Part model, mm, in its own coordinate system. Face numbers are marked on the shaded views. A direction names the side the tool comes from. Coordinates: 2 decimals unless noted, no trailing zeros. Write each loop counter-clockwise with the first axis right and the second up, starting at its lowest first coordinate (ties: lowest second). Pieces come first, ordered by that corner, then holes. Notation, with made-up numbers: (25.25, 25) -> (53.25, 25) arc R18 ccw to (53.25, 54) -> close; hole circle Ø1 at (-22, -9.75). An arc over 180 degrees is marked (long way). Write item = value, one per line.
from build123d import *

# Parameters (mm, degrees)
BOSS_EXTRUDE1_DEPTH = 50
FILLET1_R           = 10
SKETCH2_R           = 5
CUT_EXTRUDE1_DEPTH  = 170
SKETCH4_R           = 7.5
CUT_EXTRUDE2_DEPTH  = 10


with BuildPart() as part:
    # Sketch1 → Boss-Extrude1 (new body)
    with BuildSketch(Plane.XY):
        Polygon((0, 0), (0, 275), (160, 275), (160, 0), (150, 0), (150, 265), (10, 265), (10, 0), align=None)
    extrude(amount=BOSS_EXTRUDE1_DEPTH)

    # Fillet1
    fillet1_edges = [part.edges().sort_by_distance(p)[0] for p in [
        (5, 0, 0),
        (0, 275, 25),
        (160, 275, 25),
        (155, 0, 50),
        (5, 0, 50),
        (155, 0, 0),
    ]]
    fillet(fillet1_edges, radius=FILLET1_R)

    # Sketch2 → Cut-Extrude1 (cut)
    with BuildSketch(Plane.ZY):
        with Locations(Location((25, 25, 0), (0, 0, 270))):
            Circle(SKETCH2_R)
    extrude(amount=-CUT_EXTRUDE1_DEPTH, mode=Mode.SUBTRACT)

    # Sketch4 → Cut-Extrude2 (cut)
    with BuildSketch(Plane(origin=(0, 275, 0), x_dir=(1, 0, 0), z_dir=(0, 1, 0))):
        with Locations(Location((75, -25, 0), (0, 0, 270))):
            Circle(SKETCH4_R)
    extrude(amount=-CUT_EXTRUDE2_DEPTH, mode=Mode.SUBTRACT)


solid = part.part
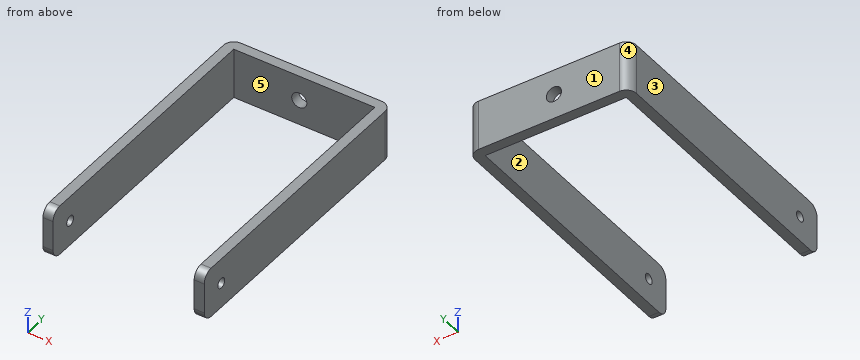
Q1. Saw through at A-A on y = 25. Give the cut face in (x, z), and give its area (3 significant figures).
Model answer:
outline = (0, 0) -> (10, 0) -> (10, 20) -> (0, 20) -> close; (0, 30) -> (10, 30) -> (10, 50) -> (0, 50) -> close; (150, 0) -> (160, 0) -> (160, 20) -> (150, 20) -> close; (150, 30) -> (160, 30) -> (160, 50) -> (150, 50) -> close
area = 800 mm²
Q2. Saw through at D-D on x = 75. Give the cut face in (y, z).
Model answer:
outline = (265, 0) -> (275, 0) -> (275, 17.5) -> (265, 17.5) -> close; (265, 32.5) -> (275, 32.5) -> (275, 50) -> (265, 50) -> close
Q3. Saw through at B-B on z = 25. Give the cut face in (x, y).
Model answer:
outline = (0, 0) -> (10, 0) -> (10, 20) -> (0, 20) -> close; (0, 30) -> (10, 30) -> (10, 265) -> (67.5, 265) -> (67.5, 275) -> (10, 275) arc R10 ccw to (0, 265) -> close; (82.5, 265) -> (150, 265) -> (150, 30) -> (160, 30) -> (160, 265) arc R10 ccw to (150, 275) -> (82.5, 275) -> close; (150, 0) -> (160, 0) -> (160, 20) -> (150, 20) -> close
Q4. Probe line 1 (X direction, y = 173, z = 13); line 2 (Z direction, x = 2, y = 25); line 3 (X direction, y = 269, z = 25). List the from-to ranges inside material, lowest first. Write a range as from..to.
Model answer:
line_1 = 0..10, 150..160
line_2 = 0..20, 30..50
line_3 = 0.83..67.5, 82.5..159.17
Q5. Pin check, flat tips, straight feed: pin 1 (3 mm diameter, centred on x = 34.5, z = 42, fed in from -Y); pin 2 (13 mm diameter, centred on y = 25, z = 25, fed in from +X). Stop position of each tip, or through.
Model answer:
pin_1 = 265
pin_2 = 160
Q6. Mould opens along X. For the marked faces 1, 2 and 3 say: released by +X, released by -X, zero draft, split by the parting line, or undercut.
Model answer:
face_1 = zero draft
face_2 = undercut
face_3 = released by -X
Q7. Which spindle directions (+Z, -Z, +X, -X, +Y, -Y) get a long thin tool onto all of the face, cutting with end or side? Do the marked faces 4 and 5. Say none if no direction does.
Model answer:
face_4 = +Z, -Z, -X, +Y
face_5 = +Z, -Z, -Y
Q8. Saw through at C-C on y = 252. Give the cut face in (x, z).
Model answer:
outline = (0, 0) -> (10, 0) -> (10, 50) -> (0, 50) -> close; (150, 0) -> (160, 0) -> (160, 50) -> (150, 50) -> close
